Geometry: see drawing. Coordinates: mm, zero at the bounding-box minimum. Give positions to 0.01 mm unless a question says otherwise; leave off trailing zeros. Order: outer loops, then holes, each group sorted by start corner. A loop starts at its lowest first (then second) coordinate and runs counter-clockwise, first axis right, second up. Notation, with made-up numbers: (45.5, 66) - (98.5, 66) arc R19 cw to (98.5, 74) - close; hole circle Ø3 at (16, 51). An arc over 180 degrees is marked (long way). Write each question's results on one line, items separated by ' | '. Start each with the question number.
Item 1: Line query: line 1 along X through (y, z) = (2.25, 14); line 2 along Y through (x, z) = (1.9, 8.75); line 3 along X through (y, z) = (11.5, 16.5). Output: solid intervals per line, ascending.
Item 2: Section D-D on y = 11.75. Output: boundary loops of the cut face in (x, z).
Item 3: Contact query for flat-ended pins moving along their axis: pin 1 Ø0.9 at (x, z) = (5.5, 12.5) entering from +Y; pin 2 Ø1 at (x, z) = (2, 18) entering from +Y. Output: stop coordinate, or through.
Item 4: Mould query, pull axis X, two halves, no side actions, for the marked faces 1 and 2. Classes: released by +X, released by -X, zero draft, split by the parting line, or undercut.
Item 5: Section C-C on x = 4.25. Output: boundary loops of the cut face in (y, z), and give its area (3 significant figures).
Item 6: Section B-B on z = 5.75. Output: boundary loops of the cut face in (x, y).
Item 7: Section A-A on y = 9. Output: boundary loops of the cut face in (x, z), and give its area (3 significant figures).
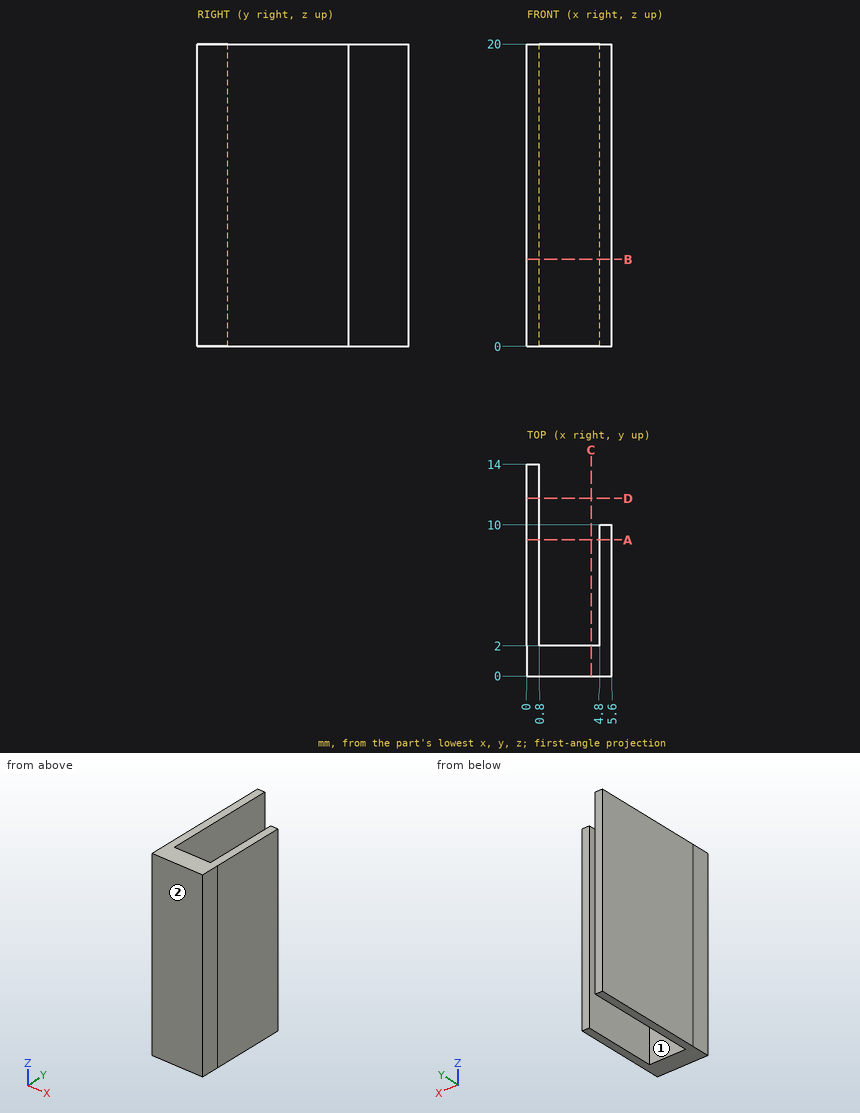
Evaluation:
1) line 1: x = 0 to 0.8, 4.8 to 5.6 | line 2: y = 0 to 2 | line 3: x = 0 to 0.8
2) outline: (0, 0) - (0.8, 0) - (0.8, 20) - (0, 20) - close
3) pin 1: stops at y = 10 | pin 2: stops at y = 2
4) face 1: undercut | face 2: zero draft
5) outline: (0, 0) - (2, 0) - (2, 20) - (0, 20) - close | area: 40.0 mm^2
6) outline: (0, 0) - (5.6, 0) - (5.6, 2) - (5.6, 10) - (4.8, 10) - (4.8, 2) - (0.8, 2) - (0.8, 14) - (0, 14) - (0, 2) - close
7) outline: (0, 0) - (0.8, 0) - (0.8, 20) - (0, 20) - close; (4.8, 0) - (5.6, 0) - (5.6, 20) - (4.8, 20) - close | area: 32.0 mm^2
